from build123d import *

# Parameters (mm, degrees)
SKETCH_1_W             = 150
SKETCH_1_H             = 8
EXTRUDE_1_DEPTH        = 10
EXTRUDE_2_DEPTH        = 10
PATTERN_LINEAR_1_COUNT = 24
PATTERN_LINEAR_1_PITCH = 6.283185307
SKETCH_3_W             = 2
SKETCH_3_H             = 1.5
CUT_EXTRUDE_1_DEPTH    = 151.545674132
SKETCH_4_W             = 32
SKETCH_4_H             = 22
SKETCH_4_R             = 5
EXTRUDE_1_2_DEPTH      = 4


with BuildPart() as part:
    # 草图1 → Extrude 1 (new body)
    with BuildSketch(Plane.XY):
        with Locations((75, -4)):
            Rectangle(SKETCH_1_W, SKETCH_1_H)
    extrude(amount=EXTRUDE_1_DEPTH)

    # 草图2 → 拉伸2 (add)
    with BuildSketch(Plane.XY.offset(10)):
        Polygon((0, 0), (1.637866054, 4.5), (3.323577771, 4.5), (4.961443825, 0), align=None)
    extrude_2 = extrude(amount=-EXTRUDE_2_DEPTH)

    # 阵列(线性)1: 拉伸2 ×24
    with Locations(*[(i * PATTERN_LINEAR_1_PITCH, 0, 0) for i in range(1, PATTERN_LINEAR_1_COUNT)]):
        add(extrude_2)

    # 草图3 → 切除-拉伸1 (cut, through all)
    with BuildSketch(Plane.ZY):
        with Locations((9, -2.25)):
            Rectangle(SKETCH_3_W, SKETCH_3_H)
        with Locations((1, -5.25)):
            Rectangle(SKETCH_3_W, SKETCH_3_H)
    extrude(amount=-CUT_EXTRUDE_1_DEPTH, mode=Mode.SUBTRACT)

    # 草图4 → Extrude 1 2 (add)
    with BuildSketch(Plane(origin=(150, 0, 0), x_dir=(0, 0, -1), z_dir=(1, 0, 0))):
        with Locations((-16, -2)):
            Rectangle(SKETCH_4_W, SKETCH_4_H)
        with Locations((-22, -2)):
            Circle(SKETCH_4_R, mode=Mode.SUBTRACT)
    extrude(amount=-EXTRUDE_1_2_DEPTH)


solid = part.part
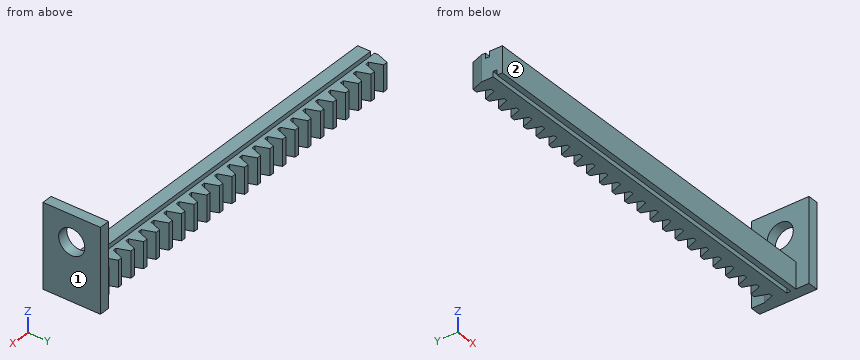
Could you check a few things on this model? Use its own coordinates, in mm. Face numbers are marked on the shaded views. A direction names the side the tool comes from. Round coordinates to 2 decimals unless told otherwise and drop trailing zeros. Order: outer loops, then holes, each group sorted by start corner. A loop starts at its lowest first (then second) coordinate and runs counter-clockwise, first axis right, second up.
Q1. Please list where these lines run through material, in increasing order: probe 1 along Y at (x, z) = (148, 22); probe 2 along Z at (x, y) = (32.5, -0.75); probe 3 along X at (y, z) = (5.25, 29.5).
Geometry says:
probe 1: y = -13 to -7, 3 to 9
probe 2: z = 0 to 10
probe 3: x = 146 to 150
Q2. Which directions (+Z, -Z, +X, -X, +Y, -Y) give clear straight access to the entire face, cutting with the end or side of a thin tool? Please do the marked faces 1 and 2.
Geometry says:
face 1: +Z, -Z, +X, +Y, -Y
face 2: +Z, -Z, -X, -Y
Q3. Imagine slicing it at A-A, the plane z = 22. List the corners of the cut face in (x, y) for me.
Geometry says:
outline: (146, -13) - (150, -13) - (150, -7) - (146, -7) - close; (146, 3) - (150, 3) - (150, 9) - (146, 9) - close
Q4. Imagine slicing it at B-B, the plane y = 1.5. State how many separate pieces and enclosed holes the cut face has, then the cut area to 3 significant figures.
Geometry says:
separate pieces: 25
enclosed holes: 0
area: 999 mm2
Q5. I'm going to push flat-ended pins straight in: P1, Ø1.3, axis at x = 116, z = 7.5, coming from the +Y side; P2, Ø2, axis at x = 77, z = 8.5, coming from the -Y side; P3, Ø8, axis at y = 5.5, z = 28, coming from the -X side. Where does each tip first touch, or does it pass through?
Geometry says:
P1: stops at y = 4.5
P2: stops at y = -8
P3: stops at x = 146
